```python
from build123d import *

# Parameters (mm, degrees)
SKETCH1_R           = 12.6365
BOSS_EXTRUDE1_DEPTH = 12.7
SKETCH2_R           = 15.875
BOSS_EXTRUDE2_DEPTH = 9.525
CHAMFER1_SIZE       = 0.4
CUT_EXTRUDE1_DEPTH  = 32.590851128


with BuildPart() as part:
    # Sketch1 → Boss-Extrude1 (new body)
    with BuildSketch(Plane(origin=(0, 0, 0), x_dir=(0, 0, -1), z_dir=(1, 0, 0))):
        Circle(SKETCH1_R)
    extrude(amount=BOSS_EXTRUDE1_DEPTH)

    # Sketch2 → Boss-Extrude2 (add)
    with BuildSketch(Plane.ZY):
        with Locations(Location((0, 0, 0), (0, 0, 180))):
            Circle(SKETCH2_R)
    extrude(amount=BOSS_EXTRUDE2_DEPTH)

    # Chamfer1
    chamfer1_edges = [part.edges().sort_by_distance(p)[0] for p in [
        (12.7, 0, 12.6365),
        (0, 0, 15.875),
        (-9.525, 0, 15.875),
    ]]
    chamfer(chamfer1_edges, length=CHAMFER1_SIZE)

    # Sketch4 → Cut-Extrude1 (cut, through all)
    with BuildSketch(Plane.ZY.offset(9.525)):
        Polygon((0, 7.332348419), (-6.35, 3.666174209), (-6.35, -3.666174209), (0, -7.332348419), (6.35, -3.666174209), (6.35, 3.666174209), align=None)
    extrude(amount=-CUT_EXTRUDE1_DEPTH, mode=Mode.SUBTRACT)


solid = part.part
```
Model file for the job. Use its own axes, mm. A direction names the side the tool comes from. Coordinates: 2 decimals unless noted, no trailing zeros. Write each loop counter-clockwise with the first axis right and the second up, starting at its lowest first coordinate (ties: lowest second). Pieces come first, ordered by that corner, then holes. Notation, with made-up numbers: (-26.75, -2) - (-0.75, -2) arc R21 ccw to (-0.75, 32) - close; hole circle Ø10 at (38, 19.25). An arc over 180 degrees is marked (long way). Use a Markdown table: item, result. Add a question column.
Item 1: Drop flat-ended pins along their axis: pin 1 (1 mm diameter, centred on y = 0.5, z = 5.5, fed in from +X); pin 2 (1.5 mm diameter, centred on x = -6.5, z = 10, fed in from +Y); pin 3 (4 mm diameter, centred on x = 2.5, y = -7, fed in from +Z); pin 4 (1.5 mm diameter, centred on x = -3.5, z = 7, fed in from +Y). Give the stop position or say it passes through.
Item 2: 3-axis set-ups, long thin cutter, end or side, ignore diameter. For faces 1 (the face through (-9.525, 0, -7)), 2 (the face through (1.432, -5.525, 3.131)), 3 (the face through (6.06, -11.21, -5.83)): which of +Z, -Z, +X, -X, +Y, -Y reach the whole face in a straight line?
Item 3: Band-saw the part on A-A, the plane x = 7. Write the cut outline in (y, z).
Item 4: Drill centre lines: line 1 along Z through (x, y) = (-2.25, -4.5); line 2 along Z through (x, y) = (8.25, -3); line 3 along Y through (x, z) = (5, -6). Where is each one in solid material? Low to high.
Item 5: Two-plate mould, pull along Y, no slides. Class faces 4 (the face through (0, 0, 13)), 5 (the face through (-4.701, 15.497, 3.441)), 6 (the face through (1, 0, 6.35)): pulls with the +Y half, pulls with the -Y half, needs draft (parallel to the pull), parting line crosses it, or undercut.
Item 6: Band-saw the part on C-C, the plane x = -6. Write the cut outline in (y, z) (3 decimals), and give its area (3 significant figures).
A:
| question | item | result |
|---|---|---|
| 1 | pin 1 | passes through |
| 1 | pin 2 | stops at y = 12.9 |
| 1 | pin 3 | stops at z = 11.61 |
| 1 | pin 4 | stops at y = 14.59 |
| 2 | face 1 | +Z, -Z, -X, +Y, -Y |
| 2 | face 2 | +X, -X |
| 2 | face 3 | +X |
| 3 | outline | circle Ø25.27 at (0, 0); hole (-7.33, 0) - (-3.67, -6.35) - (3.67, -6.35) - (7.33, 0) - (3.67, 6.35) - (-3.67, 6.35) - close |
| 4 | line 1 | z = -15.22 to -4.91, 4.91 to 15.22 |
| 4 | line 2 | z = -12.28 to -6.35, 6.35 to 12.28 |
| 4 | line 3 | y = -11.12 to -3.87, 3.87 to 11.12 |
| 5 | face 4 | needs draft |
| 5 | face 5 | parting line crosses it |
| 5 | face 6 | undercut |
| 6 | outline | circle Ø31.75 at (0, 0); hole (-7.332, 0) - (-3.666, -6.35) - (3.666, -6.35) - (7.332, 0) - (3.666, 6.35) - (-3.666, 6.35) - close |
| 6 | area | 652 mm² |
